Can you work these out from the model? Positions are in its coordinate system, mm. Give positions to 0.01 mm unless a question says otherwise; leave off trailing zeros. Loops run counter-clockwise (first coordinate to the right, second up) from the corner with the lowest first, then second, coordinate; pieces in that order, holes last. Notation, with made-up numbers: M 10.25,53.5 L 31.25,53.5 A14 ccw 31.25,71.5 Z; hole C 25.25,48 d6. An arc over 180 degrees is marked long. One line per item, written item: value. Start each with the question number.
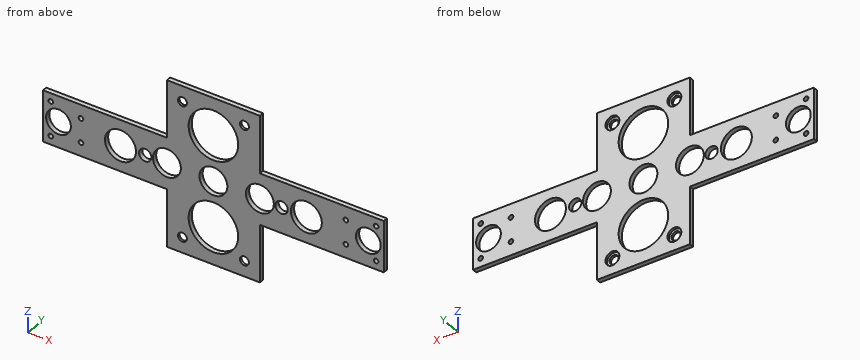
from build123d import *

# Parameters (mm, degrees)
SKETCH_1_R          = 1.5
SKETCH_1_R_2        = 9
SKETCH_1_R_3        = 8
SKETCH_1_R_4        = 10
SKETCH_1_R_5        = 2.9
SKETCH_1_R_6        = 16
SKETCH_1_R_7        = 4
EXTRUDE_1_DEPTH     = 3
SKETCH_2_R          = 4.5
CUT_EXTRUDE_1_DEPTH = 1.5


with BuildPart() as part:
    # 草图1 → 凸台-拉伸1 (new body)
    with BuildSketch(Plane(origin=(0, 0, 0), x_dir=(1, 0, 0), z_dir=(0, 1, 0))):
        Polygon((0, 0), (80, 0), (80, 37), (110, 37), (140, 37), (140, 0), (220, 0), (220, -33), (140, -33), (140, -70), (80, -70), (80, -33), (0, -33), align=None)
        with Locations((5, -27.75)):
            Circle(SKETCH_1_R, mode=Mode.SUBTRACT)
        with Locations((5, -5.45)):
            Circle(SKETCH_1_R, mode=Mode.SUBTRACT)
        with Locations((24.5, -8.7)):
            Circle(SKETCH_1_R, mode=Mode.SUBTRACT)
        with Locations((24.5, -24.3)):
            Circle(SKETCH_1_R, mode=Mode.SUBTRACT)
        with Locations((195.5, -8.7)):
            Circle(SKETCH_1_R, mode=Mode.SUBTRACT)
        with Locations((195.5, -24.3)):
            Circle(SKETCH_1_R, mode=Mode.SUBTRACT)
        with Locations((215, -27.75)):
            Circle(SKETCH_1_R, mode=Mode.SUBTRACT)
        with Locations((215, -5.45)):
            Circle(SKETCH_1_R, mode=Mode.SUBTRACT)
        with Locations((110, -16.5)):
            Circle(SKETCH_1_R_2, mode=Mode.SUBTRACT)
        with Locations((140, -16.796485685)):
            Circle(SKETCH_1_R_2, mode=Mode.SUBTRACT)
        with Locations((10, -16.5)):
            Circle(SKETCH_1_R_3, mode=Mode.SUBTRACT)
        with Locations((210, -16.5)):
            Circle(SKETCH_1_R_3, mode=Mode.SUBTRACT)
        with Locations((170, -16.5)):
            Circle(SKETCH_1_R_4, mode=Mode.SUBTRACT)
        with Locations((80, -16.796485685)):
            Circle(SKETCH_1_R_2, mode=Mode.SUBTRACT)
        with Locations((50, -16.5)):
            Circle(SKETCH_1_R_4, mode=Mode.SUBTRACT)
        with Locations((130, 27)):
            Circle(SKETCH_1_R_5, mode=Mode.SUBTRACT)
        with Locations((90, 27)):
            Circle(SKETCH_1_R_5, mode=Mode.SUBTRACT)
        with Locations((130, -60)):
            Circle(SKETCH_1_R_5, mode=Mode.SUBTRACT)
        with Locations((90, -60)):
            Circle(SKETCH_1_R_5, mode=Mode.SUBTRACT)
        with Locations((110, 13)):
            Circle(SKETCH_1_R_6, mode=Mode.SUBTRACT)
        with Locations((110, -46)):
            Circle(SKETCH_1_R_6, mode=Mode.SUBTRACT)
        with Locations((66, -16.5)):
            Circle(SKETCH_1_R_7, mode=Mode.SUBTRACT)
        with Locations((154, -16.5)):
            Circle(SKETCH_1_R_7, mode=Mode.SUBTRACT)
    extrude(amount=EXTRUDE_1_DEPTH)

    # 草图2 → 切除-拉伸1 (cut)
    with BuildSketch(Plane(origin=(0, 3, 0), x_dir=(1, 0, 0), z_dir=(0, 1, 0))):
        with Locations((90, 27)):
            Circle(SKETCH_2_R)
        with Locations((130, 27)):
            Circle(SKETCH_2_R)
        with Locations((90, -60)):
            Circle(SKETCH_2_R)
        with Locations((130, -60)):
            Circle(SKETCH_2_R)
    extrude(amount=-CUT_EXTRUDE_1_DEPTH, mode=Mode.SUBTRACT)


solid = part.part
Q1. If we section it at B-B, the plane z = 46: Write out the boundary of the cut face in (x, y), plus the area to 3 significant figures.
Q2. I need wall thicknesses on line 1 along Z through (x, y) = (90, 1.1); line 2 along X through (y, z) = (1.5, 46); line 3 along Z through (x, y) = (10, 1.4). Which ranges of each line are inside material? Lowest first, please.
Q3. If we section it at D-D, the plane y = 0.9: Give the number of separate pieces and of enclosed holes in the cut face, plus the area to 3 significant figures.
Q4. For P1, Ø4, axis at x = 195.5, z = 8.7, coming from the +Y side; P2, Ø1.5, axis at y = 1.5, z = -14, coming from the -X side; P3, Ø8, axis at x = 130, z = 60, coming from the +Y side, each with a flat end and sliding along its axis, tell me the tip position at first contact or that it passes through.
Q5. If we section it at A-A, the plane x = 170: Write out the boundary of the cut face in (y, z), plus the area to 3 significant figures.
Q6. If we section it at C-C, the plane x = 114: Write out the boundary of the cut face in (y, z), plus the area to 3 significant figures.
Response:
1. outline: M 80,0 L 94,0 L 94,3 L 80,3 Z; M 126,0 L 140,0 L 140,3 L 126,3 Z
1. area: 84.0 mm^2
2. line 1: -37 to -29.9, -24.1 to 57.1, 62.9 to 70
2. line 2: 80 to 94, 126 to 140
2. line 3: 0 to 8.5, 24.5 to 33
3. separate pieces: 1
3. enclosed holes: 23
3. area: 8,030 mm^2
4. P1: y = 3
4. P2: x = 80
4. P3: y = 1.5
5. outline: M 0,0 L 3,0 L 3,6.5 L 0,6.5 Z; M 0,26.5 L 3,26.5 L 3,33 L 0,33 Z
5. area: 39.0 mm^2
6. outline: M 0,-37 L 3,-37 L 3,-28.49 L 0,-28.49 Z; M 0,2.49 L 3,2.49 L 3,8.44 L 0,8.44 Z; M 0,24.56 L 3,24.56 L 3,30.51 L 0,30.51 Z; M 0,61.49 L 3,61.49 L 3,70 L 0,70 Z
6. area: 86.7 mm^2
